Autodesk Inventor part; units mm, degrees
ref_plane "YZ Plane" through (0, 0, 0) normal (1, 0, 0) x (0, 1, 0)
ref_plane "XZ Plane" through (0, 0, 0) normal (0, 1, 0) x (-1, 0, 0)
ref_plane "XY Plane" through (0, 0, 0) normal (0, 0, 1) x (1, 0, 0)
sketch "Sketch1" plane through (0, 0, 0) normal (0, 1, 0) x (-1, 0, 0)
  line L0 (132.0119, -3.8652) -> (-67.9881, -3.8652)
  line L1 (-67.9881, -3.8652) -> (-67.9881, 5.1348)
  line L2 (-67.9881, 5.1348) -> (132.0119, 5.1348)
  line L3 (132.0119, 5.1348) -> (132.0119, -3.8652)
  point P0 (0, 0)
  dimension "d0" = 200
  dimension "d1" = 9
extrude "Extrusion1" add sketch "Sketch1" along normal blind 6.5
sketch "Sketch2" plane through (0, 6.5, 0) normal (0, 1, 0) x (1, 0, 0)
  circle A0 centre (57.9881, -0.6348) radius 1.75
  line L0 (67.9881, 3.8652) -> (-132.0119, 3.8652)
  line L1 (67.9881, -5.1348) -> (67.9881, 3.8652)
  circle A1 centre (37.9881, -0.6348) radius 1.75
  circle A2 centre (17.9881, -0.6348) radius 1.75
  circle A3 centre (-2.0119, -0.6348) radius 1.75
  circle A4 centre (-22.0119, -0.6348) radius 1.75
  circle A5 centre (-42.0119, -0.6348) radius 1.75
  circle A6 centre (-62.0119, -0.6348) radius 1.75
  circle A7 centre (-82.0119, -0.6348) radius 1.75
  circle A8 centre (-102.0119, -0.6348) radius 1.75
  circle A9 centre (-122.0119, -0.6348) radius 1.75
  point P0 (0, 0)
  dimension "d4" = 3.5
  dimension "d5" = 4.5
  dimension "d6" = 10
  dimension "d9" = 20
extrude "Extrusion2" cut sketch "Sketch2" against normal through all
properties part number "MGN9x200mm_rail"
Source: CAD feature listing. Evaluate the final solid. Frame: model axes, mm. Round coordinates to 2 decimals unless told otherwise and drop trailing zeros. Answer as a JSON object with one key per item and string values. Group by question number.
Q1. Section query A-A (y = 1). State how many separate pieces and enclosed holes the cut face has, plus the area to 3 significant figures.
Q2. Mould query, pull axis Z, two halves, no side actions, for faces 1 (the flat face through (-31, 3, 5.135)), 2 (the cylindrical face through (-20.343, 3.296, 0.109)), 3 (the flat face through (-31, 0, 1)). Classes: pulls with the +Z half, pulls with the -Z half, needs draft (parallel to the pull), parting line crosses it, or undercut.
Q3. Ray query, line 1 (Z direction, x = 58, y = 0.5); line 2 (Z direction, x = -101, y = 2). Return the intervals inside material, ascending. Write a range as from..to.
Completed:
{
 "1": {"separate pieces": "1", "enclosed holes": "10", "area": "1,700 mm²"},
 "2": {"face 1": "pulls with the +Z half", "face 2": "undercut", "face 3": "needs draft"},
 "3": {"line 1": "-3.87..-1.12, 2.38..5.13", "line 2": "-3.87..-0.79, 2.06..5.13"}
}
